For this review, use the dimensioned drawing (mm, ordinates from the lowest corner) and the shaded views. Give positions to 0.01 mm unless a question says otherwise; leave off trailing zeros. Order: outer loops, then holes, each group sorted by start corner. A loop starts at its lowest first (then second) coordinate and runs counter-clockwise, first axis right, second up.
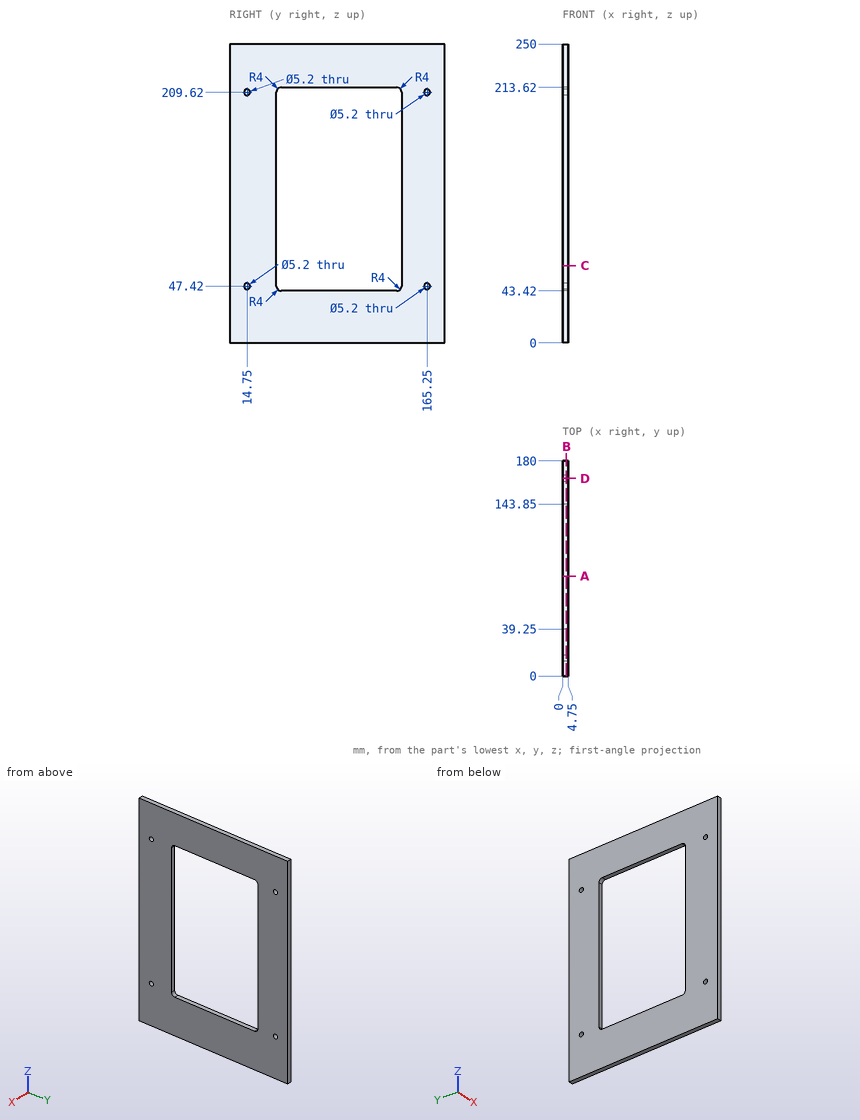
1. Take a section at C-C (z = 64.5). State the section outline as (x, y) points.
Recorded:
outline: (0, 0) - (4.75, 0) - (4.75, 39.25) - (0, 39.25) - close; (0, 143.85) - (4.75, 143.85) - (4.75, 180) - (0, 180) - close
2. For pin 1 (12 mm diameter, centred on y = 36, z = 97.5, fed in from -X); pin 2 (3 mm diameter, centred on y = 14.75, z = 47.42, fed in from +X), all flat-tipped, find the tip position at first contact; note any pin that passes through.
Recorded:
pin 1: stops at x = 0
pin 2: passes through
3. Take a section at B-B (x = 3). State the section outline as (y, z) points.
Recorded:
outline: (0, 0) - (180, 0) - (180, 250) - (0, 250) - close; hole circle Ø5.2 at (14.75, 47.42); hole circle Ø5.2 at (14.75, 209.62); hole (39.25, 47.42) arc R4 ccw to (43.25, 43.42) - (139.85, 43.42) arc R4 ccw to (143.85, 47.42) - (143.85, 209.62) arc R4 ccw to (139.85, 213.62) - (43.25, 213.62) arc R4 ccw to (39.25, 209.62) - close; hole circle Ø5.2 at (165.25, 47.42); hole circle Ø5.2 at (165.25, 209.62)
4. Take a section at A-A (y = 83.5). State the section outline as (x, z) points, then the cut area to 3 significant figures.
Recorded:
outline: (0, 0) - (4.75, 0) - (4.75, 43.42) - (0, 43.42) - close; (0, 213.62) - (4.75, 213.62) - (4.75, 250) - (0, 250) - close
area: 379 mm2
5. For line 1 along Z through (x, y) = (2.1, 14.75); line 2 along Y through (x, z) = (1.35, 209.62); line 3 along Y through (x, z) = (2.35, 69), list the stretches that pass through material, from the lowest coordinate up.
Recorded:
line 1: z = 0 to 44.82, 50.02 to 207.02, 212.22 to 250
line 2: y = 0 to 12.15, 17.35 to 39.25, 143.85 to 162.65, 167.85 to 180
line 3: y = 0 to 39.25, 143.85 to 180
6. Take a section at D-D (y = 165.25). State the section outline as (x, z) points, then the cut area to 3 significant figures.
Recorded:
outline: (0, 0) - (4.75, 0) - (4.75, 44.82) - (0, 44.82) - close; (0, 50.02) - (4.75, 50.02) - (4.75, 207.02) - (0, 207.02) - close; (0, 212.22) - (4.75, 212.22) - (4.75, 250) - (0, 250) - close
area: 1,140 mm2
